For this review, take the finished solid that the model builds, in its own axes (mm). Give positions to 0.01 mm unless a question says otherwise; leave off trailing zeros. Order: outer loops, then holes, each group sorted by start corner. A loop starts at its lowest first (then second) coordinate and runs counter-clockwise, first axis right, second up.
from build123d import *

# Parameters (mm, degrees)
F0_R     = 27.400357
F2_DEPTH = 1.778
F1_R     = 17.246114
F3_DEPTH = 1.778
F5_R     = 1.152069
F6_DEPTH = 8.89
F7_COUNT = 5


with BuildPart() as f2:
    # F0 (on Top) → F2 (new body)
    with BuildSketch(Plane.XY):
        Circle(F0_R)
    extrude(amount=F2_DEPTH)

    # F1 (on Top) → F3 (cut, through all)
    with BuildSketch(Plane.XY):
        Circle(F1_R)
    extrude(amount=F3_DEPTH, mode=Mode.SUBTRACT)


with BuildPart() as f6:
    # F5 (on Top) → F6 (new body, symmetric)
    with BuildSketch(Plane.XY):
        with Locations((0, 19.281207)):
            Circle(F5_R)
    extrude(amount=F6_DEPTH, both=True)


with BuildPart() as f7_1:
    # F7: instance of F6
    add(f6.part.rotate(Axis((0, 0, 1.187779), (0, 0, -1)), 1 * 360 / F7_COUNT))


with BuildPart() as f7_2:
    # F7: instance of F6
    add(f6.part.rotate(Axis((0, 0, 1.187779), (0, 0, -1)), 2 * 360 / F7_COUNT))


with BuildPart() as f7_3:
    # F7: instance of F6
    add(f6.part.rotate(Axis((0, 0, 1.187779), (0, 0, -1)), 3 * 360 / F7_COUNT))


with BuildPart() as f7_4:
    # F7: instance of F6
    add(f6.part.rotate(Axis((0, 0, 1.187779), (0, 0, -1)), 4 * 360 / F7_COUNT))


with BuildPart() as f2_1:
    add(f2.part)

    # F8: cut F7_4, F6, F7_1, F7_2, F7_3
    add(f7_4.part, mode=Mode.SUBTRACT)
    add(f6.part, mode=Mode.SUBTRACT)
    add(f7_1.part, mode=Mode.SUBTRACT)
    add(f7_2.part, mode=Mode.SUBTRACT)
    add(f7_3.part, mode=Mode.SUBTRACT)


solid = f2_1.part
1) To check wall thickness, follow line 1 (Y direction, x = 0, z = 1.2); line 2 (Y direction, x = -1, z = 0.3); line 3 (X direction, y = -16, z = 0.95). State the ranges of each line that lie inside material, in increasing order.
Answer sheet:
line 1: y = -27.4 to -17.25, 17.25 to 18.13, 20.43 to 27.4
line 2: y = -27.38 to -17.22, 17.22 to 18.71, 19.85 to 27.38
line 3: x = -22.24 to -12.41, -10.25 to -6.44, 6.44 to 10.25, 12.41 to 22.24
2) We need section D-D on z = 1.15. Give the boundary of the cut face in (x, y).
Answer sheet:
outline: circle Ø54.8 at (0, 0); hole circle Ø2.3 at (-18.34, 5.96); hole circle Ø34.49 at (0, 0); hole circle Ø2.3 at (-11.33, -15.6); hole circle Ø2.3 at (0, 19.28); hole circle Ø2.3 at (11.33, -15.6); hole circle Ø2.3 at (18.34, 5.96)
3) We need section B-B on y = 0. Give the boundary of the cut face in (x, z).
Answer sheet:
outline: (-27.4, 0) - (-17.25, 0) - (-17.25, 1.78) - (-27.4, 1.78) - close; (17.25, 0) - (27.4, 0) - (27.4, 1.78) - (17.25, 1.78) - close
4) Draft analysis for pull direction X (two halves, no side actions). For faces 1 (the face through (0, -18, 0)), 2 (the face through (19.453, 5.669, 0.901)), 3 (the face through (-20.195, 18.518, 0.877)), state which applies: +X half, -X half, draft (parallel to the pull), parting line (faces both ways), or undercut.
Answer sheet:
face 1: draft
face 2: undercut
face 3: parting line
5) Clearance check with flat-ended pins moving along their axes: pin 1 (1.4 mm diameter, centred on x = -18.34, y = 5.96, fed in from +Z); pin 2 (1 mm diameter, centred on y = 4, z = 1, fed in from +X). State where each tip first meets the part, or that it passes through.
Answer sheet:
pin 1: passes through
pin 2: stops at x = 27.18
6) We need section C-C on x = 7.5. Give the boundary of the cut face in (y, z).
Answer sheet:
outline: (-26.35, 0) - (-15.53, 0) - (-15.53, 1.78) - (-26.35, 1.78) - close; (15.53, 0) - (26.35, 0) - (26.35, 1.78) - (15.53, 1.78) - close
7) We need section A-A on x = 0. Give the boundary of the cut face in (y, z), then the cut area to 3 significant figures.
Answer sheet:
outline: (-27.4, 0) - (-17.25, 0) - (-17.25, 1.78) - (-27.4, 1.78) - close; (17.25, 0) - (18.13, 0) - (18.13, 1.78) - (17.25, 1.78) - close; (20.43, 0) - (27.4, 0) - (27.4, 1.78) - (20.43, 1.78) - close
area: 32.0 mm2
